The drawing under review shows one solid part. Ordinate dimensions are in mm from its lowest x, y, z. A direction names the side the tool comes from. Coordinates: 2 decimals unless noted, no trailing zeros. Write each loop counter-clockwise with the first axis right and the second up, starting at its lowest first coordinate (ties: lowest second). Pieces come first, ordered by that corner, then holes.
1) Add section C-C, the plane x = 55.5. State the section outline as (y, z) points, then the cut area to 3 significant figures.
2) Add section B-B, the plane y = 55. State the section outline as (x, z) points.
3) Machinability: for the marked faces 5, 6, 7, 8 and 9, which of the approach directions +Z, -Z, +X, -X, +Y, -Y give a long, thin tool a straight path to every point of the face, cutting with its end or side? Answer none if there is none.
4) For line 1 (X direction, y = 27.5, z = 8); line 2 (X direction, y = 64, z = 14); line 3 (X direction, y = 42.5, z = 19.5), list the stretches that pass through material, from the lowest coordinate up.
5) Add section D-D, the plane z = 47. State the section outline as (x, y) points.
6) For P1, Ø3, axis at y = 45.5, z = 41, coming from the -X side; P2, Ø21, axis at y = 54.5, z = 11, coming from the +X side; P3, Ø7.5, axis at x = 137.5, y = 68.5, coming from the +Z side, all flat-tipped, find the tip position at first contact; note any pin that passes through.
7) Mouldability with a two-part tool opening along X and no side actions: class the marked faces 1, 2, 3 and 4 as released by +X, released by -X, zero draft, split by the parting line, or undercut.
8) Add section A-A, the plane z = 17. State the section outline as (x, y) points.
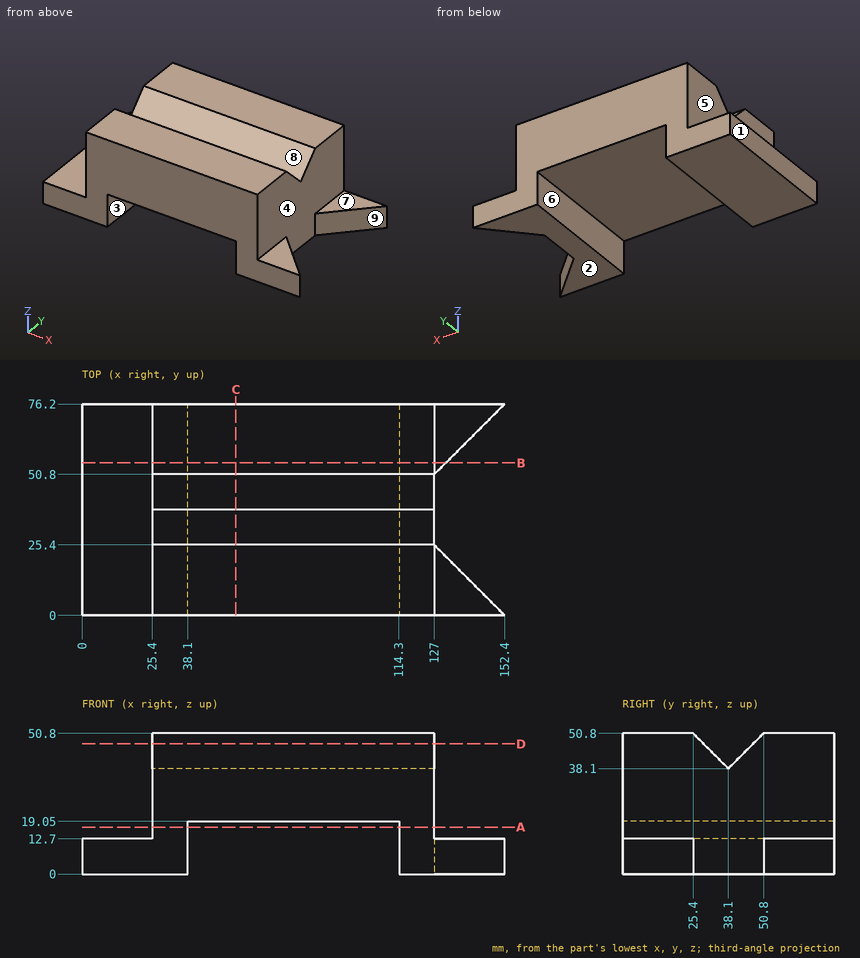
Geometry results:
1. outline: (0, 19.05) - (76.2, 19.05) - (76.2, 50.8) - (50.8, 50.8) - (38.1, 38.1) - (25.4, 50.8) - (0, 50.8) - close
1. area: 2,260 mm2
2. outline: (0, 0) - (38.1, 0) - (38.1, 19.05) - (114.3, 19.05) - (114.3, 0) - (131.2, 0) - (131.2, 12.7) - (127, 12.7) - (127, 50.8) - (25.4, 50.8) - (25.4, 12.7) - (0, 12.7) - close
3. face 5: +Z, -X, +Y, -Y
3. face 6: -Z, +Y, -Y
3. face 7: +Z, +X, +Y, -Y
3. face 8: +Z, +X, -X
3. face 9: +Z, -Z, +X
4. line 1: x = 0 to 38.1, 114.3 to 127
4. line 2: x = 25.4 to 38.1, 114.3 to 127
4. line 3: x = 25.4 to 127
5. outline: (25.4, 0) - (127, 0) - (127, 29.2) - (25.4, 29.2) - close; (25.4, 47) - (127, 47) - (127, 76.2) - (25.4, 76.2) - close
6. P1: stops at x = 25.4
6. P2: stops at x = 141.2
6. P3: stops at z = 12.7
7. face 1: released by -X
7. face 2: zero draft
7. face 3: undercut
7. face 4: released by +X
8. outline: (25.4, 0) - (38.1, 0) - (38.1, 76.2) - (25.4, 76.2) - close; (114.3, 0) - (127, 0) - (127, 76.2) - (114.3, 76.2) - close
